from build123d import *

# Parameters (mm, degrees)
SKETCH_1_W          = 95.3
SKETCH_1_H          = 48
EXTRUDE_1_DEPTH     = 25
EXTRUDE_2_DEPTH     = 45
CUT_EXTRUDE_1_DEPTH = 77.619335027
CUT_EXTRUDE_2_DEPTH = 2
SKETCH_5_R          = 1.35
EXTRUDE_3_DEPTH     = 2
FILLET_1_R          = 2
FILLET_2_R          = 3
SKETCH_6_R          = 3.2
EXTRUDE_4_DEPTH     = 6
SKETCH_7_W          = 13
SKETCH_7_H          = 7.14
SKETCH_7_W_2        = 6.3
SKETCH_7_H_2        = 9.4
CUT_EXTRUDE_3_DEPTH = 5


with BuildPart() as part:
    # 草图1 → 凸台-拉伸1 (new body)
    with BuildSketch(Plane(origin=(0, 0, 0), x_dir=(1, 0, 0), z_dir=(0, 1, 0))):
        Rectangle(SKETCH_1_W, SKETCH_1_H)
    extrude(amount=EXTRUDE_1_DEPTH)

    # 草图2 → 凸台-拉伸2 (add)
    with BuildSketch(Plane(origin=(47.65, 0, 0), x_dir=(0, 0, -1), z_dir=(1, 0, 0))):
        Polygon((-24, 25), (24, 25), (24, 36), (14, 36), (14, 27.5), (-14, 27.5), (-14, 36), (-24, 36), align=None)
    extrude(amount=-EXTRUDE_2_DEPTH)

    # 草图3 → 切除-拉伸1 (cut, through all)
    with BuildSketch(Plane.XY.offset(24)):
        Polygon((2.65, 25), (2.65, 36), (9.65, 36), align=None)
        Polygon((47.65, 25), (47.65, 36), (25.15, 36), align=None)
    extrude(amount=-CUT_EXTRUDE_1_DEPTH, mode=Mode.SUBTRACT)

    # 草图4 → 切除-拉伸2 (cut)
    with BuildSketch(Plane(origin=(47.65, 0, 0), x_dir=(0, 0, -1), z_dir=(1, 0, 0))):
        with BuildLine():
            Line((-12, 22), (12, 22))
            ThreePointArc((12, 22), (13.414213562, 21.414213562), (14, 20))
            Line((14, 20), (14, 5))
            ThreePointArc((14, 5), (13.414213562, 3.585786438), (12, 3))
            Line((12, 3), (-12, 3))
            ThreePointArc((-12, 3), (-13.414213562, 3.585786438), (-14, 5))
            Line((-14, 5), (-14, 20))
            ThreePointArc((-14, 20), (-13.414213562, 21.414213562), (-12, 22))
        make_face()
    extrude(amount=-CUT_EXTRUDE_2_DEPTH, mode=Mode.SUBTRACT)

    # 草图5 → 凸台-拉伸3 (add)
    # profile 1 of 2: a face of its own
    with BuildSketch(Plane.XZ):
        Polygon((29.185898385, 24), (32.65, 30), (38.65, 30), (42.114101615, 24), align=None)
        with Locations(Location((35.65, 27, 0), (0, 0, 270))):
            Circle(SKETCH_5_R, mode=Mode.SUBTRACT)
    # profile 2 of 2: a face of its own
    with BuildSketch(Plane.XZ):
        Polygon((-42.814101615, 24), (-39.35, 30), (-33.35, 30), (-29.885898385, 24), align=None)
        with Locations(Location((-36.35, 27, 0), (0, 0, 270))):
            Circle(SKETCH_5_R, mode=Mode.SUBTRACT)
    extrude_3 = extrude(amount=-EXTRUDE_3_DEPTH)

    # 镜向1: 凸台-拉伸3 across plane
    add(extrude_3.mirror(Plane.XY))

    # 圆角1
    fillet_1_edges = [part.edges().sort_by_distance(p)[0] for p in [
        (-29.885898385, 1, 24),
        (-42.814101615, 1, 24),
        (-39.35, 1, 30),
        (-33.35, 1, 30),
        (29.185898385, 1, -24),
        (42.114101615, 1, -24),
        (38.65, 1, -30),
        (32.65, 1, -30),
        (-42.814101615, 1, -24),
        (-29.885898385, 1, -24),
        (-33.35, 1, -30),
        (-39.35, 1, -30),
        (42.114101615, 1, 24),
        (29.185898385, 1, 24),
        (32.65, 1, 30),
        (38.65, 1, 30),
    ]]
    fillet(fillet_1_edges, radius=FILLET_1_R)

    # 圆角2
    fillet_2_edges = [part.edges().sort_by_distance(p)[0] for p in [
        (2.65, 25, 0),
        (17.4, 36, -24),
        (17.4, 36, -14),
        (17.4, 36, 14),
        (17.4, 36, 24),
        (47.65, 12.5, 24),
        (47.65, 12.5, -24),
        (-47.65, 12.5, 24),
        (-47.65, 12.5, -24),
    ]]
    fillet(fillet_2_edges, radius=FILLET_2_R)

    # 草图6 → 凸台-拉伸4 (add)
    with BuildSketch(Plane.ZY.offset(47.65)):
        with Locations(Location((-7, 5.783019787, 0), (0, 0, 180))):
            Circle(SKETCH_6_R)
        with Locations(Location((7, 5.783019787, 0), (0, 0, 180))):
            Circle(SKETCH_6_R)
    extrude(amount=EXTRUDE_4_DEPTH)

    # 草图7 → 切除-拉伸3 (cut)
    with BuildSketch(Plane.XY.offset(24)):
        with Locations((-9.15, 11.158)):
            Rectangle(SKETCH_7_W, SKETCH_7_H)
        with Locations((-37.16, 17.87)):
            Rectangle(SKETCH_7_W_2, SKETCH_7_H_2)
    extrude(amount=-CUT_EXTRUDE_3_DEPTH, mode=Mode.SUBTRACT)


solid = part.part
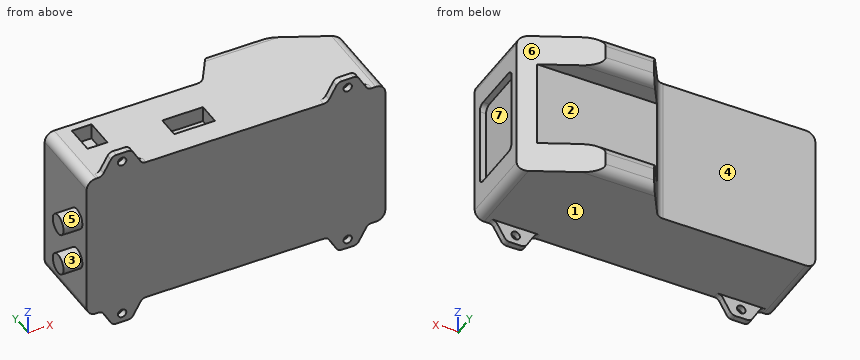
CAD build for the part. Positions are in the model's coordinates, mm. Face numbers are marked on the shaded views. A direction names the side the tool comes from. Round coordinates to 2 decimals unless told otherwise and drop trailing zeros. Loops run counter-clockwise (first coordinate to the right, second up) from the corner with the lowest first, then second, coordinate; pieces in that order, holes last. Notation, with made-up numbers: M -8.75,53.25 L 23.25,53.25 A20 ccw 23.25,57.25 Z; hole C 17,53 d2. An arc over 180 degrees is marked long. One line per question, with ' | ' between items. Start each with the question number.
Item 1: Pin check, flat tips, straight feed: pin 1 Ø5 at (x, z) = (38, 27.5) entering from +Y; pin 2 Ø6 at (y, z) = (27.5, -16.5) entering from +X; pin 3 Ø14 at (x, z) = (19.5, 4.5) entering from +Y; pin 4 Ø1.5 at (y, z) = (18.5, 21.5) entering from -X. Stop position of each tip, or through.
Item 2: Cut at B-B, the plane z = 1.5. Write the cut outline in (x, y), plus the area to 3 significant figures.
Item 3: Wall check: line 1 (Y direction, x = -12, z = 20.5); line 2 (Z direction, x = 21, y = 30.5); line 3 (X direction, y = 1, z = 27). Give the ranges that are in metal, low to high.
Item 4: Cut at A-A, the plane x = -36.35. Write the cut outline in (y, z).
Item 5: Cut at D-D, the plane x = 21.5. Write the cut outline in (y, z).
Item 6: Which spindle directions (+Z, -Z, +X, -X, +Y, -Y) get a long thin tool onto all of the face, cutting with end or side? Do the marked faces 5, 6 and 7. Say none if no direction does.
Item 7: Two-plate mould, pull along Z, no slides. Class the marked faces 1, 2, 3 and 4: pulls with the +Z half, pulls with the -Z half, needs draft (parallel to the pull), parting line crosses it, or undercut.
Item 8: Cut at C-C, the plane z = 27. Write the cut outline in (x, y), plus the area to 3 significant figures.
Responses:
1) pin 1: stops at y = 2 | pin 2: stops at x = 47.65 | pin 3: stops at y = 27.5 | pin 4: stops at x = -47.65
2) outline: M -47.65,0 L 47.65,0 L 47.65,3 L 45.65,3 L 45.65,22 L 47.65,22 L 47.65,25 L 42.54,27.5 L 4.24,27.5 L 3.53,26.39 A3 cw 1,25 L -47.65,25 Z | area: 2,450 mm²
3) line 1: y = 0 to 7.59, 14.73 to 25 | line 2: z = -24 to -14, 14 to 24 | line 3: x = -41.08 to -37.7, -35 to -31.62, 30.92 to 34.3, 37 to 40.38
4) outline: M 0,-30 L 2,-30 L 2,-28.35 L 0,-28.35 Z; M 0,-25.65 L 2,-25.65 L 2,-24 L 25,-24 L 25,24 L 22.57,24 L 22.57,19 L 13.17,19 L 13.17,24 L 2,24 L 2,25.65 L 0,25.65 Z; M 0,28.35 L 2,28.35 L 2,30 L 0,30 Z
5) outline: M 0,-24 L 33,-24 A3 ccw 36,-21 L 36,-17 A3 ccw 33,-14 L 27.5,-14 L 27.5,14 L 33,14 A3 ccw 36,17 L 36,21 A3 ccw 33,24 L 0,24 Z
6) face 5: -X | face 6: +Z, -Z, +X, +Y | face 7: +X
7) face 1: pulls with the -Z half | face 2: undercut | face 3: undercut | face 4: needs draft
8) outline: M -41.08,0 L -37.7,0 L -37.7,2 L -41.08,2 Z; M -35,0 L -31.62,0 L -31.62,2 L -35,2 Z; M 30.92,0 L 34.3,0 L 34.3,2 L 30.92,2 Z; M 37,0 L 40.38,0 L 40.38,2 L 37,2 Z | area: 27.1 mm²
